```python
from build123d import *

# Parameters (mm, degrees)
F1_DEPTH = 100
F3_DEPTH = 30
F4_R     = 5


with BuildPart() as f1:
    # F0 (on Top) → F1 (new body)
    with BuildSketch(Plane.XY):
        with BuildLine():
            Line((0, 50), (0, 0))
            Line((0, 0), (100, 0))
            ThreePointArc((100, 0), (114.6446609407, 35.3553390593), (150, 50))
            Line((150, 50), (150, 150))
            Line((150, 150), (70, 150))
            Line((70, 150), (0, 50))
        make_face()
    extrude(amount=F1_DEPTH)

    # F2 (on face) → F3 (cut)
    with BuildSketch(Plane.XY.offset(100)):
        with BuildLine():
            Line((20, 43.6955553836), (20, 20))
            Line((20, 20), (82.917960675, 20))
            ThreePointArc((82.917960675, 20), (100.5025253169, 49.4974746831), (130, 67.082039325))
            Line((130, 67.082039325), (130, 130))
            Line((130, 130), (80.4131112315, 130))
            Line((80.4131112315, 130), (20, 43.6955553836))
        make_face()
    extrude(amount=-F3_DEPTH, mode=Mode.SUBTRACT)

    # F4
    f4_edges = [f1.edges().sort_by_distance(p)[0] for p in [
        (20, 31.847778, 70),
        (51.45898, 20, 70),
        (100.502525, 49.497475, 70),
        (130, 98.54102, 70),
        (105.206556, 130, 70),
        (50.206556, 86.847778, 70),
        (80.413111, 130, 85),
        (20, 43.695555, 85),
        (50.206556, 86.847778, 100),
        (82.917961, 20, 85),
        (130, 67.082039, 85),
        (100.502525, 49.497475, 100),
        (20, 20, 85),
        (20, 31.847778, 100),
        (130, 130, 85),
        (130, 98.54102, 100),
        (105.206556, 130, 100),
        (51.45898, 20, 100),
    ]]
    fillet(f4_edges, radius=F4_R)


solid = f1.part
```
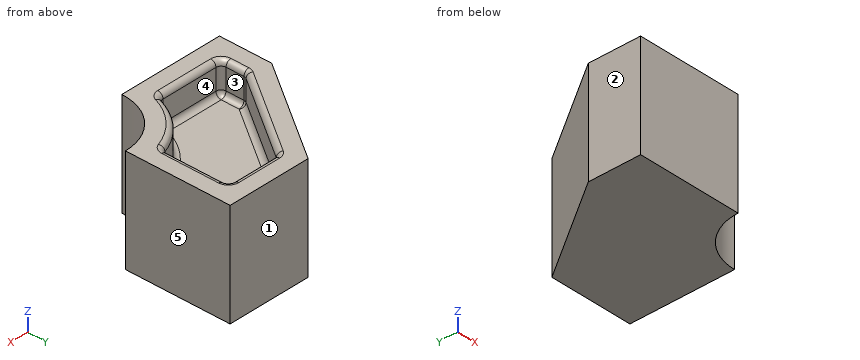
Read the model definition and answer for the solid it produces. Units are mm, in the model's axes. Face numbers are marked on the shaded views. A direction names the side the tool comes from. Give positions to 0.01 mm unless a question says otherwise; leave off trailing zeros. Loops run counter-clockwise (first coordinate to the right, second up) from the corner with the lowest first, then second, coordinate; pieces in that order, holes last.
Item 1: Each of these flat-tipped pins is pushed along its axis until it touches: pin 1 Ø1.5 at (y, z) = (134.5, 19.5) entering from -X (3 decimals); pin 2 Ø3 at (x, y) = (70.5, 25.5) entering from +Z; pin 3 Ø22 at (y, z) = (99.5, 80.5) entering from -X. Where does it stop, or does it pass through?
Item 2: For the marked faces 4 and 5, determine the directions among +Z, -Z, +X, -X, +Y, -Y from which every point of the face is accessible in a straight line to the end or side of a thin tool.
Item 3: The part is cut by section B-B (z = 61). Write down the section's boundary in (x, y), and give its area (3 significant figures).
Item 4: The part is cut by section A-A (z = 88). Write down the section's boundary in (x, y).
Item 5: The part is cut by section C-C (x = 10). Write down the section's boundary in (y, z).
Item 6: The mould has two halves that part along Y. Classify the marked faces 1, 2 and 3: released by +Y, released by -Y, zero draft, split by the parting line, or undercut.
Item 7: Find the intervals of material crossed by line 1 along Z through (x, y) = (92, 92); line 2 along Y through (x, z) = (35, 43); line 3 along Y through (x, z) = (28, 72.5), in increasing order.
Taken from the geometry:
1. pin 1: stops at x = 58.625
1. pin 2: stops at z = 70.1
1. pin 3: stops at x = 26.95
2. face 4: +Z
2. face 5: +Z, -Z, +X, +Y, -Y
3. outline: (0, 0) - (100, 0) arc R50 cw to (150, 50) - (150, 150) - (70, 150) - (0, 50) - close
3. area: 17,000 mm2
4. outline: (0, 0) - (100, 0) arc R50 cw to (150, 50) - (150, 150) - (70, 150) - (0, 50) - close; hole (20, 25) arc R5 ccw to (25, 20) - (79.29, 20) arc R5 ccw to (84, 23.33) arc R70 cw to (126.67, 66) arc R5 ccw to (130, 70.71) - (130, 125) arc R5 ccw to (125, 130) - (83.02, 130) arc R5 ccw to (78.92, 127.87) - (20.9, 44.99) arc R5 ccw to (20, 42.12) - close
5. outline: (0, 0) - (64.29, 0) - (64.29, 100) - (0, 100) - close
6. face 1: released by +Y
6. face 2: zero draft
6. face 3: undercut
7. line 1: z = 0 to 70
7. line 2: y = 0 to 100
7. line 3: y = 0 to 20.67, 53.96 to 90
